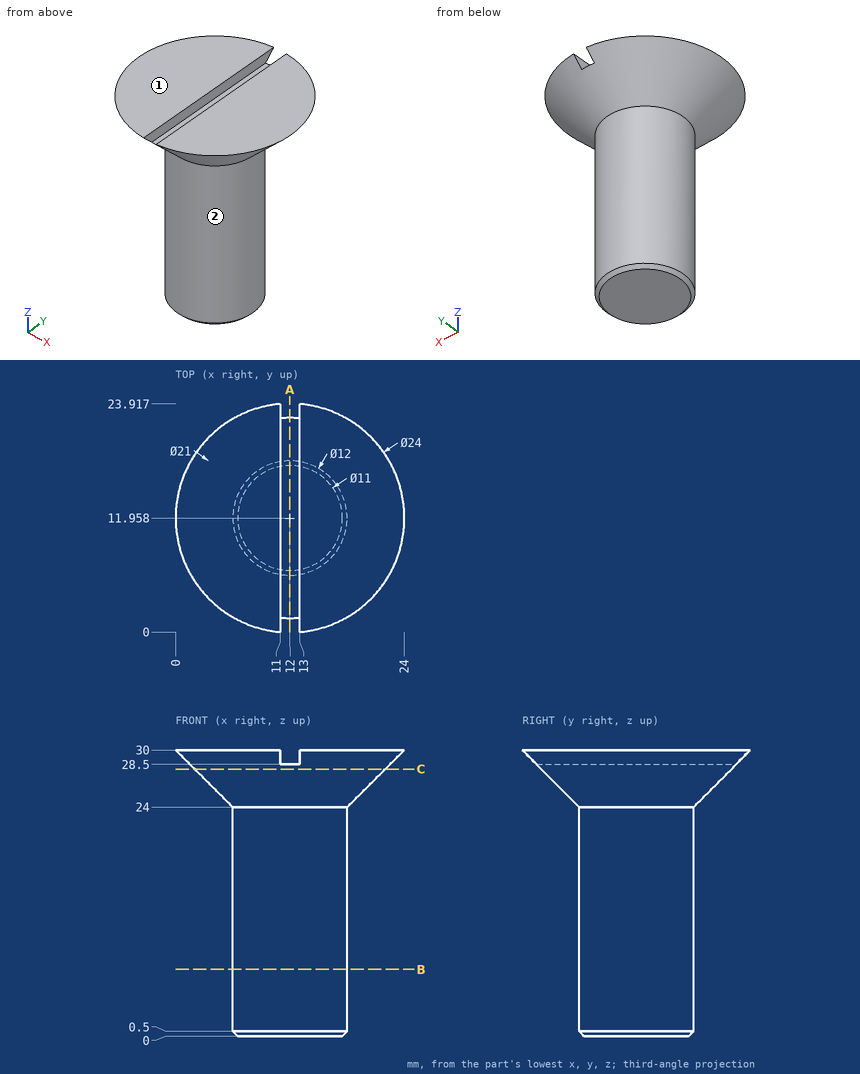
Here's the drawing with two shaded views (mm, measured from the low corner). I have some questions. A direction names the side the tool comes from. Coordinates: 2 decimals unless noted, no trailing zeros. Loops run counter-clockwise (first coordinate to the right, second up) from the corner with the lowest first, then second, coordinate; pieces in that order, holes last. Notation, with made-up numbers: (-35, -1) -> (15, -1) arc R5 cw to (15, 6) -> close; hole circle Ø5 at (-6, 69.5). An arc over 180 degrees is marked (long way). Put each result on its own line as item: value. Start each with the question number.
Q1. For the marked faces 1 and 2, which set-ups out of +Z, -Z, +X, -X, +Y, -Y let a thin tool reach every point of the face, with its end or its side?
Q2. I want a section at C-C (z = 28). Write out the boundary of the cut face in (x, y).
Q3. I want a section at B-B (z = 7). Write out the boundary of the cut face in (x, y).
Q4. If I drill on line 1 (Z direction, x = 12.5, y = 17); line 2 (Y direction, x = 16, z = 6) (1 decimal); line 3 (Y direction, x = 9.25, z = 23) (1 decimal), over which ranges is the centre line in solid material (lowest first)? Write a range as [from, to].
Q5. I'm going to push flat-ended pins straight in: P1, Ø1.2, axis at y = 15.5, z = 29.5, coming from the -X side; P2, Ø10, axis at y = 19.5, z = 5.5, coming from the -X side (1 decimal); P3, Ø1.5, axis at x = 10.5, z = 20, coming from the +Y side. Where does each tip first touch, or does it pass through?
Q6. I want a section at A-A (x = 12). Write out the boundary of the cut face in (y, z), plus the area to 3 significant figures.
Taken from the geometry:
1. face 1: +Z, +X, -X, +Y, -Y
1. face 2: -Z
2. outline: circle Ø20 at (12, 11.96)
3. outline: circle Ø12 at (12, 11.96)
4. line 1: z = [0, 28.5]
4. line 2: y = [7.5, 16.4]
4. line 3: y = [6.6, 17.3]
5. P1: stops at x = 0.44
5. P2: stops at x = 6.6
5. P3: stops at y = 17.91
6. outline: (1.46, 28.5) -> (5.96, 24) -> (5.96, 0.5) -> (6.46, 0) -> (17.46, 0) -> (17.96, 0.5) -> (17.96, 24) -> (22.46, 28.5) -> close
6. area: 362 mm2
